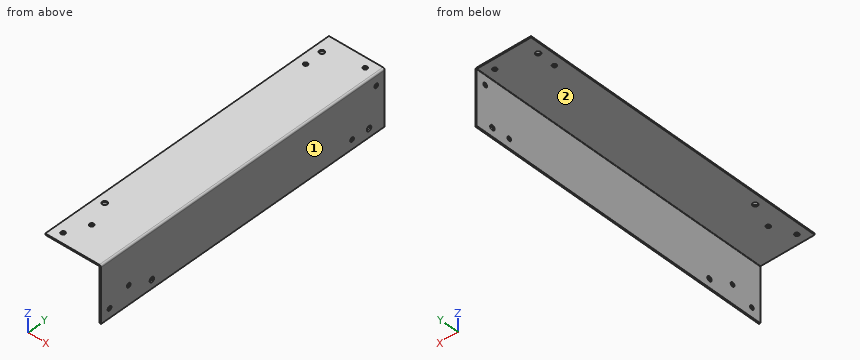
from build123d import *

# Parameters (mm, degrees)
SKETCH1_W                    = 60
SKETCH1_H                    = 334.61392
BASE_FLANGE1_DEPTH           = 1.51892
EDGE_FLANGE1_STRIP_W         = 6.83768
EDGE_FLANGE1_STRIP_H         = 1.51892
EDGE_FLANGE1_STRIP_CUT_DEPTH = 334.61392
EDGE_FLANGE1_DEPTH           = 334.61392
M5_CLEARANCE_HOLE1_D         = 5.3
M5_CLEARANCE_HOLE2_D         = 5.3
M4_CLEARANCE_HOLE1_D         = 4.5
M4_CLEARANCE_HOLE2_D         = 4.5


# Sheet-metal steps are written as plain solids
with BuildPart() as part:
    # Sketch1 → Base-Flange1 (new body)
    with BuildSketch(Plane(origin=(0, 0, 0), x_dir=(0, 0, -1), z_dir=(1, 0, 0))):
        with Locations((-30, 167.30696)):
            Rectangle(SKETCH1_W, SKETCH1_H)
    extrude(amount=-BASE_FLANGE1_DEPTH)

    # Edge-Flange1 strip (across the edge) → Edge-Flange1 strip cut (cut)
    with BuildSketch(Plane(origin=(-1.51892, 0, 60), x_dir=(0, 0, -1), z_dir=(0, 1, 0))):
        with Locations((-1.51892, -0.75946)):
            Rectangle(EDGE_FLANGE1_STRIP_W, EDGE_FLANGE1_STRIP_H)
    extrude(amount=EDGE_FLANGE1_STRIP_CUT_DEPTH, mode=Mode.SUBTRACT)

    # Edge-Flange1 section (across the edge) → Edge-Flange1 (add)
    with BuildSketch(Plane(origin=(-1.51892, 0, 60), x_dir=(0, 0, -1), z_dir=(0, 1, 0))):
        with BuildLine():
            Line((0, 0.381), (0, 58.48108))
            Line((0, 58.48108), (1.51892, 58.48108))
            Line((1.51892, 58.48108), (1.51892, 0.381))
            ThreePointArc((1.51892, 0.381), (1.630512316, 0.111592316), (1.89992, 0))
            Line((1.89992, 0), (1.89992, -1.51892))
            ThreePointArc((1.89992, -1.51892), (0.556473684, -0.962446316), (0, 0.381))
        make_face()
    extrude(amount=EDGE_FLANGE1_DEPTH)

    # M5 Clearance Hole1 (through all)
    with Locations(Plane.XY.offset(60)):
        with Locations((-50.726027, 60), (-50.726027, 316.13284)):
            Hole(M5_CLEARANCE_HOLE1_D / 2)

    # M5 Clearance Hole2 (through all)
    with Locations(Plane(origin=(0, 0, 0), x_dir=(0, 0, -1), z_dir=(1, 0, 0))):
        with Locations((-9.273973, 60), (-9.273973, 316.13284)):
            Hole(M5_CLEARANCE_HOLE2_D / 2)

    # M4 Clearance Hole1 (through all)
    with Locations(Plane.XY.offset(60)):
        with Locations((-50, 296.13284), (-11.89992, 324.61392), (-50, 10), (-40, 32.714)):
            Hole(M4_CLEARANCE_HOLE1_D / 2)

    # M4 Clearance Hole2 (through all)
    with Locations(Plane(origin=(0, 0, 0), x_dir=(0, 0, -1), z_dir=(1, 0, 0))):
        with Locations((-10, 296.13284), (-48.10008, 324.61392), (-10, 10), (-20, 32.714)):
            Hole(M4_CLEARANCE_HOLE2_D / 2)


solid = part.part
The listing builds one solid part. Answer for the finished solid, in the listing's coordinates (mm). Face numbers are marked on the shaded views. A direction names the side the tool comes from. Give positions to 0.01 mm unless a question says otherwise; leave off trailing zeros. Write each loop counter-clockwise with the first axis right and the second up, starting at its lowest first coordinate (ties: lowest second). Pieces come first, ordered by that corner, then holes. Notation, with made-up numbers: (-27.75, 57.5) -> (6.25, 57.5) arc R27 ccw to (6.25, 90.5) -> close; hole circle Ø8 at (22, -22). An arc over 180 degrees is marked (long way). One line per question, with ' | ' between items. Start each with the question number.
1. Section A-A (y = 162.5) is taken. Determine the outline of the cut face in (x, z).
2. Find the intervals of material crossed by probe 1 along Y at (x, z) = (-0.6, 10); probe 2 along Y at (x, z) = (-40, 59); probe 3 along Z at (x, y) = (-17.5, 100.5), in increasing order.
3. Section B-B (z = 41.5) is taken. Determine the outline of the cut face in (x, y), plus the area to 3 significant figures.
4. Section C-C (x = -32) is taken. Determine the outline of the cut face in (y, z).
5. Given pin 1 Ø3 at (y, z) = (135, 53.5) entering from -X; pin 2 Ø5 at (x, y) = (-45.5, 176.5) entering from -Z, each flat-ended and moving along its own axis, determine where each tip first touches the part or whether it passes through.
6. For the marked faces 1 and 2, determine the directions among +Z, -Z, +X, -X, +Y, -Y from which every point of the face is accessible in a straight line to the end or side of a thin tool.
Response values:
1) outline: (-60, 58.48) -> (-1.9, 58.48) arc R0.38 cw to (-1.52, 58.1) -> (-1.52, 0) -> (0, 0) -> (0, 58.1) arc R1.9 ccw to (-1.9, 60) -> (-60, 60) -> close
2) probe 1: 0 to 7.75, 12.25 to 57.45, 62.55 to 293.88, 298.38 to 313.58, 318.68 to 334.61 | probe 2: 0 to 30.46, 34.96 to 334.61 | probe 3: 58.48 to 60
3) outline: (-1.52, 0) -> (0, 0) -> (0, 334.61) -> (-1.52, 334.61) -> close | area: 508 mm2
4) outline: (0, 58.48) -> (334.61, 58.48) -> (334.61, 60) -> (0, 60) -> close
5) pin 1: x = -1.52 | pin 2: z = 58.48
6) face 1: +Z, -Z, +X, +Y, -Y | face 2: -Z, -X, +Y, -Y
